Can you work these out from the drawing? Everything is in mm from the part's minimum corner. A direction names the side the tool comes from. Give positions to 0.01 mm unless a question says otherwise; leave off trailing zeros. Write each loop counter-clockwise with the first axis right and the second up, starting at its lowest first coordinate (ties: lowest second). Pieces come first, ordered by that corner, then holes. Notation, with made-up numbers: (6, -28) -> (61, -28) arc R20 cw to (61, -10) -> close; hole circle Ø7 at (14.5, 71). An arc over 180 degrees is marked (long way). Use one line per item in the form item = value.
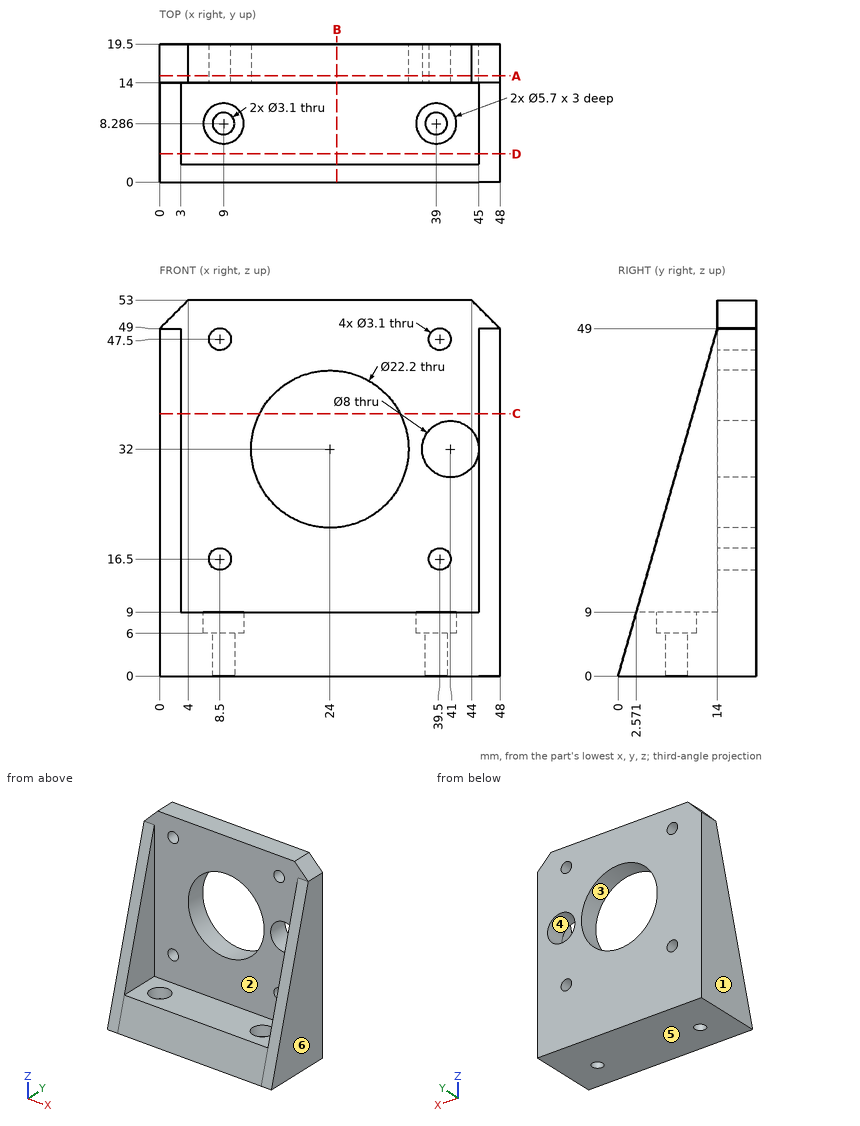
Q1. If I drill on line 1 along X through (y, z) = (18, 16.5); line 2 along X through (y, z) = (18.75, 32); line 3 along Z through (x, y) = (8.5, 17.1), over which ranges is the centre line in solid material (lowest first)? Write a range as from..to.
Result set:
line_1 = 0..6.95, 10.05..37.95, 41.05..48
line_2 = 0..12.9, 35.1..37, 45..48
line_3 = 0..14.95, 18.05..45.95, 49.05..53
Q2. I want a section at B-B, the plane x = 25. Write out the boundary of the cut face in (y, z) (1 decimal).
Result set:
outline = (0, 0) -> (19.5, 0) -> (19.5, 20.9) -> (14, 20.9) -> (14, 9) -> (2.6, 9) -> close; (14, 43.1) -> (19.5, 43.1) -> (19.5, 53) -> (14, 53) -> close
Q3. I want a section at C-C, the plane z = 37. Write out the boundary of the cut face in (x, y).
Result set:
outline = (0, 10.57) -> (3, 10.57) -> (3, 14) -> (14.09, 14) -> (14.09, 19.5) -> (0, 19.5) -> close; (33.91, 14) -> (45, 14) -> (45, 10.57) -> (48, 10.57) -> (48, 19.5) -> (33.91, 19.5) -> close
Q4. I want a section at A-A, the plane y = 15. Write out the boundary of the cut face in (x, z).
Result set:
outline = (0, 0) -> (48, 0) -> (48, 49) -> (44, 53) -> (4, 53) -> (0, 49) -> close; hole circle Ø3.1 at (8.5, 16.5); hole circle Ø3.1 at (8.5, 47.5); hole circle Ø22.2 at (24, 32); hole circle Ø8 at (41, 32); hole circle Ø3.1 at (39.5, 16.5); hole circle Ø3.1 at (39.5, 47.5)
Q5. I want a section at D-D, the plane y = 4. Write out the boundary of the cut face in (x, z).
Result set:
outline = (0, 0) -> (48, 0) -> (48, 14) -> (45, 14) -> (45, 9) -> (3, 9) -> (3, 14) -> (0, 14) -> close
Q6. If we mould it in two halves opening along Z, with no side actions, what happens to the marked faces 3, 4, 5 and 6? For each: +Z half, -Z half, draft (parallel to the pull), parting line (faces both ways), or undercut.
Result set:
face_3 = undercut
face_4 = undercut
face_5 = -Z half
face_6 = draft
Q7. Which directions (+Z, -Z, +X, -X, +Y, -Y) give clear straight access to the entire face, cutting with the end or side of a thin tool? Please do the marked faces 1 and 2.
Result set:
face_1 = +Z, -Z, -X, +Y, -Y
face_2 = +Z, -Y
Q8. Will these pins go through, and if not, where does the flat tip stop? pin 1 Ø6.5 at (x, y) = (10, 9.5) entering from +Z; pin 2 Ø3.5 at (x, y) = (39, 8.29) entering from +Z; pin 3 Ø22 at (x, z) = (27.5, 29.5) entering from -Y.
Result set:
pin_1 = 9
pin_2 = 6
pin_3 = 14
